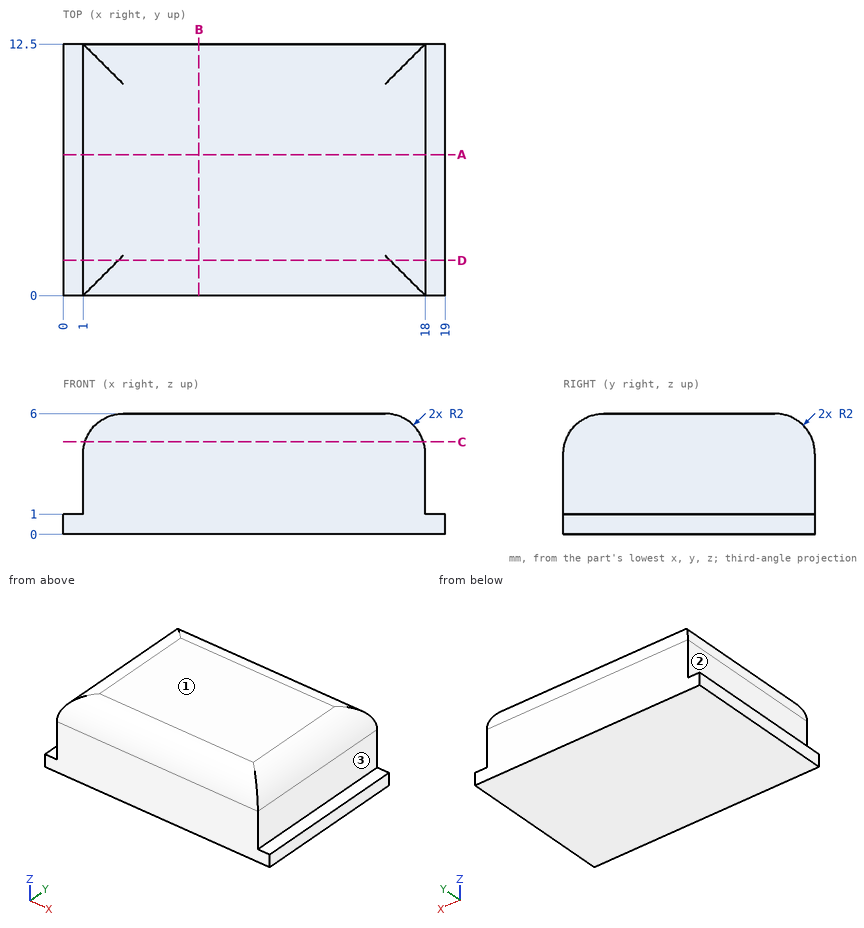
For this review, use the dimensioned drawing (mm, ordinates from the lowest corner) and the shaded views. A direction names the side the tool comes from. Give positions to 0.01 mm unless a question says otherwise; leave off trailing zeros. Order: outer loops, then holes, each group sorted by start corner. A loop starts at its lowest first (then second) coordinate and runs counter-clockwise, first axis right, second up. Notation, with made-up numbers: (35, 44.25) - (85, 44.25) arc R28 ccw to (85, 71.25) - close; hole circle Ø11 at (68, 10.5). An arc over 180 degrees is marked (long way). Use CSV: the item, a comma, the result in double quotes. Start each with the question number.
Q1. Take a section at C-C (z = 4.6). State the section outline as (x, y) points, and give its area (3 significant figures).
Q2. Take a section at D-D (y = 1.75). State the section outline as (x, z) points.
Q3. Take a section at B-B (x = 6.75). State the section outline as (y, z) points, and give its area (3 significant figures).
Q4. For P1, Ø6, axis at x = 10.5, y = 6, coming from the -Z side; P2, Ø3, axis at y = 2, z = 4.5, coming from the +X side; P3, Ø0.5, axis at x = 0.5, y = 8, coming from the +Z side, all flat-tipped, find the tip position at first contact; note any pin that passes through.
Q5. For line 1 (X direction, y = 1.5, z = 2.1); line 2 (Z direction, x = 7, y = 11.25); line 3 (X direction, y = 9.75, z = 5.05), list the stretches that pass through material, from the lowest coordinate up.
Q6. Take a section at A-A (y = 7). State the section outline as (x, z) points.
Q7. Machinability: for the marked faces 1, 2 and 3, which of the approach directions +Z, -Z, +X, -X, +Y, -Y give a long, thin tool a straight path to every point of the face, cutting with its end or side? Answer none if there is none.
Calculated:
1,outline,"(1.09, 0.09) - (17.91, 0.09) - (17.91, 12.41) - (1.09, 12.41) - close"
1,area,"207 mm²"
2,outline,"(0, 0) - (19, 0) - (19, 1) - (18, 1) - (18, 4) arc R2 ccw to (16.25, 5.98) - (2.75, 5.98) arc R2 ccw to (1, 4) - (1, 1) - (0, 1) - close"
3,outline,"(0, 0) - (12.5, 0) - (12.5, 4) arc R2 ccw to (10.5, 6) - (2, 6) arc R2 ccw to (0, 4) - close"
3,area,"73.3 mm²"
4,P1,"stops at z = 0"
4,P2,"stops at x = 18"
4,P3,"stops at z = 1"
5,line 1,"x = 1 to 18"
5,line 2,"z = 0 to 5.85"
5,line 3,"x = 1.3 to 17.7"
6,outline,"(0, 0) - (19, 0) - (19, 1) - (18, 1) - (18, 4) arc R2 ccw to (16, 6) - (3, 6) arc R2 ccw to (1, 4) - (1, 1) - (0, 1) - close"
7,face 1,"+Z, +X, -X, +Y, -Y"
7,face 2,"+Z, -X, +Y, -Y"
7,face 3,"+Z, +X, +Y, -Y"
